The listing builds one solid part. Answer for the finished solid, in the listing's coordinates (mm). A direction names the side the tool comes from. Give positions to 0.01 mm unless a question says otherwise; leave off trailing zeros. Order: outer loops, then holes, each group sorted by start corner. A loop starts at its lowest first (then second) coordinate and runs counter-clockwise, first axis right, second up. Notation, with made-up numbers: (31.25, -16.5) - (58.25, -16.5) arc R14 ccw to (58.25, -1.5) - close; hole circle Ø7 at (83, -4.5). An arc over 180 degrees is marked (long way). Answer in a Markdown table with one row per item. Add a question column.
```python
from build123d import *

# Parameters (mm, degrees)
SKETCH1_W           = 120
SKETCH1_H           = 50
BOSS_EXTRUDE1_DEPTH = 160
FILLET1_R           = 5
FILLET2_R           = 5
SKETCH2_W           = 100
SKETCH2_H           = 140
CUT_EXTRUDE1_DEPTH  = 45
FILLET3_R           = 5
FILLET4_R           = 5
FILLET5_R           = 5
SKETCH3_R           = 1.5
CUT_EXTRUDE2_DEPTH  = 20
SKETCH4_W           = 70
SKETCH4_H           = 27
CUT_EXTRUDE4_DEPTH  = 20


with BuildPart() as part:
    # Sketch1 → Boss-Extrude1 (new body)
    with BuildSketch(Plane.XY):
        with Locations((60, -25)):
            Rectangle(SKETCH1_W, SKETCH1_H)
    extrude(amount=BOSS_EXTRUDE1_DEPTH)

    # Fillet1
    fillet1_edges = [part.edges().sort_by_distance(p)[0] for p in [
        (0, -25, 160),
    ]]
    fillet(fillet1_edges, radius=FILLET1_R)

    # Fillet2
    fillet2_edges = [part.edges().sort_by_distance(p)[0] for p in [
        (120, -25, 160),
        (120, -25, 0),
        (0, -25, 0),
    ]]
    fillet(fillet2_edges, radius=FILLET2_R)

    # Sketch2 → Cut-Extrude1 (cut)
    with BuildSketch(Plane.XZ.offset(50)):
        with Locations((60, 80)):
            Rectangle(SKETCH2_W, SKETCH2_H)
    extrude(amount=-CUT_EXTRUDE1_DEPTH, mode=Mode.SUBTRACT)

    # Fillet3
    fillet3_edges = [part.edges().sort_by_distance(p)[0] for p in [
        (10, -27.5, 10),
        (10, -27.5, 150),
        (110, -27.5, 150),
        (110, -27.5, 10),
    ]]
    fillet(fillet3_edges, radius=FILLET3_R)

    # Fillet4
    fillet4_edges = [part.edges().sort_by_distance(p)[0] for p in [
        (110, -5, 80),
        (60, -5, 10),
        (10, -5, 80),
        (60, -5, 150),
        (11.464466094, -5, 148.535533906),
        (108.535533906, -5, 148.535533906),
        (11.464466094, -5, 11.464466094),
        (108.535533906, -5, 11.464466094),
    ]]
    fillet(fillet4_edges, radius=FILLET4_R)

    # Fillet5
    fillet5_edges = [part.edges().sort_by_distance(p)[0] for p in [
        (0, 0, 80),
        (1.464466094, 0, 158.535533906),
        (60, 0, 0),
        (60, 0, 160),
        (120, 0, 80),
        (118.535533906, 0, 158.535533906),
        (118.535533906, 0, 1.464466094),
        (1.464466094, 0, 1.464466094),
    ]]
    fillet(fillet5_edges, radius=FILLET5_R)

    # Sketch3 → Cut-Extrude2 (cut)
    with BuildSketch(Plane.XZ.offset(50)):
        with Locations((5, 155)):
            Circle(SKETCH3_R)
        with Locations((115, 155)):
            Circle(SKETCH3_R)
        with Locations((115, 5)):
            Circle(SKETCH3_R)
        with Locations((5, 5)):
            Circle(SKETCH3_R)
    extrude(amount=-CUT_EXTRUDE2_DEPTH, mode=Mode.SUBTRACT)

    # Sketch4 → Cut-Extrude4 (cut)
    with BuildSketch(Plane.XY.offset(160)):
        with Locations((60, -30.5)):
            Rectangle(SKETCH4_W, SKETCH4_H)
    extrude(amount=-CUT_EXTRUDE4_DEPTH, mode=Mode.SUBTRACT)


solid = part.part
```
(1) The mould has two halves that part along Z. Classify faces 4 (the face through (59, -5, 81)), 5 (the face through (1, -2, 81)), 6 (the face through (1, -27, 2)): +Z half, -Z half, draft (parallel to the pull), parting line (faces both ways), or undercut.
(2) Straight lines are drawn through the part: line 1 (Z direction, x = 5, y = -38.25); line 2 (X direction, y = -39.5, z = 155); line 3 (X direction, y = -21.5, z = 121.5). For each, find the intervals that lie inside material, in ascending order.
(3) Each of these flat-tipped pins is pushed along its axis until it touches: P1, Ø8, axis at x = 44.5, y = -38.5, coming from the +Z side; P2, Ø3.5, axis at x = 114.5, z = 4.5, coming from the -Y side; P3, Ø1.5, axis at x = 83.5, z = 51, coming from the -Y side; P4, Ø2.5, axis at x = 5, z = 155, coming from the -Y side. Where does it stop, or does it pass through?
(4) For faces 1 (the face through (60, -44, 155)), 2 (the face through (11, -7, 79)), 3 (the face through (59, -12, 160)), determine the directions among +Z, -Z, +X, -X, +Y, -Y from which every point of the face is accessible in a straight line to the end or side of a thin tool.
(5) Find section A-A, the plane x = 33. Write down the section's boundary in (y, z).
(6) Find section B-B, the plane y = -25.5. Write down the section's boundary in (x, z), plus the area to 3 significant figures.
(7) Find section C-C, the plane z = 50. Write down the section's boundary in (x, y).
(8) Find section D-D, the plane y = -8. Write down the section's boundary in (x, z), plus the area to 3 significant figures.
Answer key:
| question | item | result |
|---|---|---|
| 1 | face 4 | undercut |
| 1 | face 5 | draft |
| 1 | face 6 | -Z half |
| 2 | line 1 | 0 to 3.5, 6.5 to 153.5, 156.5 to 160 |
| 2 | line 2 | 0 to 3.5, 6.5 to 25, 95 to 113.5, 116.5 to 120 |
| 2 | line 3 | 0 to 10, 110 to 120 |
| 3 | P1 | z = 10 |
| 3 | P2 | y = -50 |
| 3 | P3 | y = -5 |
| 3 | P4 | y = -30 |
| 4 | face 1 | +Z |
| 4 | face 2 | -Y |
| 4 | face 3 | +Z, +X, -X, +Y, -Y |
| 5 | outline | (-50, 0) - (-5, 0) arc R5 ccw to (0, 5) - (0, 155) arc R5 ccw to (-5, 160) - (-17, 160) - (-17, 150) - (-10, 150) arc R5 cw to (-5, 145) - (-5, 15) arc R5 cw to (-10, 10) - (-50, 10) - close; (-50, 150) - (-44, 150) - (-44, 160) - (-50, 160) - close |
| 6 | outline | (0, 5) arc R5 ccw to (5, 0) - (115, 0) arc R5 ccw to (120, 5) - (120, 155) arc R5 ccw to (115, 160) - (95, 160) - (95, 150) - (105, 150) arc R5 cw to (110, 145) - (110, 15) arc R5 cw to (105, 10) - (15, 10) arc R5 cw to (10, 15) - (10, 145) arc R5 cw to (15, 150) - (25, 150) - (25, 160) - (5, 160) arc R5 ccw to (0, 155) - close |
| 6 | area | 4,500 mm² |
| 7 | outline | (0, -50) - (10, -50) - (10, -10) arc R5 cw to (15, -5) - (105, -5) arc R5 cw to (110, -10) - (110, -50) - (120, -50) - (120, -5) arc R5 ccw to (115, 0) - (5, 0) arc R5 ccw to (0, -5) - close |
| 8 | outline | (0, 5) arc R5 ccw to (5, 0) - (115, 0) arc R5 ccw to (120, 5) - (120, 155) arc R5 ccw to (115, 160) - (5, 160) arc R5 ccw to (0, 155) - close; hole (10.42, 15) arc R4.58 ccw to (15, 10.42) - (105, 10.42) arc R4.58 ccw to (109.58, 15) - (109.58, 145) arc R4.58 ccw to (105, 149.58) - (15, 149.58) arc R4.58 ccw to (10.42, 145) - close |
| 8 | area | 5,400 mm² |
